Part model, mm, in its own coordinate system. A direction names the side the tool comes from. Coordinates: 2 decimals unless noted, no trailing zeros. Order: outer loops, then holes, each group sorted by start corner. A loop starts at its lowest first (then second) coordinate and runs counter-clockwise, first axis right, second up.
1) Wall check: L1, parallel to X at y = -16.5, z = 0.55; L2, parallel to Z at x = -7.5, y = -7; L3, parallel to X at y = -5, z = 3.15. Give the ranges that are in metal, low to high.
2) Cut at C-C (z = 5.15). List the corners of the cut face in (x, y), and give its area (3 significant figures).
3) Tool access for faces 5 (the flat face through (-20, 8, 4)), 6 (the cylindrical face through (8.557, -17.126, 1.972)): list every direction of +Z, -Z, +X, -X, +Y, -Y with a clear straight run to the whole face (end or side of a thin tool).
4) Mould opens along X. For faces 1 (the cylindrical face through (-19.463, 13.212, 1.972)), 2 (the flat face through (15.3, -18.8, 2)), 3 (the flat face through (-16, 2, 6)), 4 (the cylindrical face through (-19.463, -17.788, 1.972)) say: +X half, -X half, draft (parallel to the pull), parting line (faces both ways), or undercut.
5) Cut at D-D (x = 13). List the corners of the cut face in (y, z), and give its area (3 significant figures).
6) Pin check, flat tips, straight feed: pin 1 Ø9 at (x, y) = (-2.5, -5.5) entering from +Z; pin 2 Ø5 at (x, y) = (10.11, -17.19) entering from +Z; pin 3 Ø5 at (x, y) = (-5.39, -1.69) entering from -Z; pin 4 Ø2 at (x, z) = (-6.5, 5.5) entering from +Y. Stop position of each tip, or through.
7) Cut at A-A (z = 0.8). List the corners of the cut face in (x, y).
8) Cut at B-B (x = -20.5). Give the number of separate pieces and of enclosed holes in the cut face, and give its area (3 significant figures).
```python
from build123d import *

# Parameters (mm, degrees)
F0_R     = 1.55
F0_R_2   = 16.5
F0_R_3   = 11.0000000003
F0_R_4   = 4.1499999994
F1_DEPTH = 4
F2_R     = 16.5
F2_R_2   = 11.0000000003
F3_DEPTH = 2
F4_SIZE  = 1.99999
F5_SIZE  = 1.99999


# Not quite as in the source:
# - a fillet or chamfer is up to 0.001 mm smaller than in the source, because OpenCascade refuses the exact size


with BuildPart() as f1:
    # F0 (on Top) → F1 (new body)
    with BuildSketch(Plane.XY):
        Polygon((10.9770673246, 19.3054056901), (-5.3945055504, 19.3054056901), (-21.7660784254, 19.3054056904), (-23.1802919884, 18.7196192521), (-25.8087191127, 16.0911921274), (-26.3945055504, 14.6769785651), (-26.3945055504, -18.0661671849), (-25.8087191127, -19.4803807472), (-23.1802919884, -22.1088078719), (-21.7660784254, -22.6945943101), (-5.3945055504, -22.6945943099), (10.9770673246, -22.6945943084), (12.3912808869, -22.1088078705), (15.0197080109, -19.4803807465), (15.6054944488, -18.0661671842), (15.6054944488, 14.6769785659), (15.0197080109, 16.0911921281), (12.3912808869, 18.7196192521), align=None)
        with Locations((-20.8945055404, -17.1945943099)):
            Circle(F0_R, mode=Mode.SUBTRACT)
        with Locations((-5.3945055504, -1.6945943099)):
            Circle(F0_R_2, mode=Mode.SUBTRACT)
        with Locations((10.1054944396, -17.1945943099)):
            Circle(F0_R, mode=Mode.SUBTRACT)
        with Locations((-20.8945055501, 13.8054056901)):
            Circle(F0_R, mode=Mode.SUBTRACT)
        with Locations((10.1054944396, 13.8054056901)):
            Circle(F0_R, mode=Mode.SUBTRACT)
        with Locations((-5.3945055504, -1.6945943099)):
            Circle(F0_R_2)
        with Locations((-5.3945055504, -1.6945943099)):
            Circle(F0_R_3, mode=Mode.SUBTRACT)
        with Locations((-5.3945055504, -1.6945943099)):
            Circle(F0_R_3)
        with Locations((-5.3945055504, -1.6945943099)):
            Circle(F0_R_4, mode=Mode.SUBTRACT)
    extrude(amount=F1_DEPTH)

    # F2 (on face) → F3 (join)
    with BuildSketch(Plane.XY.offset(4)):
        with Locations((-5.3945055504, -1.6945943099)):
            Circle(F2_R)
        with Locations((-5.3945055504, -1.6945943099)):
            Circle(F2_R_2, mode=Mode.SUBTRACT)
    extrude(amount=F3_DEPTH)

    # F4 (size 2 in the source; OpenCascade refuses exactly that, so slightly less here)
    f4_edges = [f1.edges().sort_by_distance(p)[0] for p in [
        (-21.894506, -1.694594, 6),
    ]]
    chamfer(f4_edges, length=F4_SIZE)

    # F5 (size 2 in the source; OpenCascade refuses exactly that, so slightly less here)
    f5_edges = [f1.edges().sort_by_distance(p)[0] for p in [
        (-16.394506, -1.694594, 4),
    ]]
    chamfer(f5_edges, length=F5_SIZE)


solid = f1.part
```
Geometry check:
1. L1: x = -26.39 to -22.28, -19.51 to 8.72, 11.49 to 15.61
1. L2: z = 0 to 4
1. L3: x = -26.39 to -7.9, -2.89 to 15.61
2. outline: circle Ø30.7 at (-5.39, -1.69); hole circle Ø20.3 at (-5.39, -1.69)
2. area: 417 mm2
3. face 5: +Z
3. face 6: +Z, -Z
4. face 1: undercut
4. face 2: +X half
4. face 3: draft
4. face 4: undercut
5. outline: (-21.5, 0) - (18.11, 0) - (18.11, 4) - (-21.5, 4) - close
5. area: 158 mm2
6. pin 1: stops at z = 4.28
6. pin 2: stops at z = 4
6. pin 3: passes through
6. pin 4: stops at y = 14.27
7. outline: (-26.39, -18.07) - (-25.81, -19.48) - (-23.18, -22.11) - (-21.77, -22.69) - (10.98, -22.69) - (12.39, -22.11) - (15.02, -19.48) - (15.61, -18.07) - (15.61, 14.68) - (15.02, 16.09) - (12.39, 18.72) - (10.98, 19.31) - (-21.77, 19.31) - (-23.18, 18.72) - (-25.81, 16.09) - (-26.39, 14.68) - close; hole circle Ø3.1 at (-20.89, -17.19); hole circle Ø3.1 at (-20.89, 13.81); hole circle Ø8.3 at (-5.39, -1.69); hole circle Ø3.1 at (10.11, -17.19); hole circle Ø3.1 at (10.11, 13.81)
8. separate pieces: 3
8. enclosed holes: 0
8. area: 156 mm2
